```python
from build123d import *

# Parameters (mm, degrees)
SKETCH1_W           = 18.5
SKETCH1_H           = 40
BOSS_EXTRUDE1_DEPTH = 3
SKETCH2_W           = 1.5
SKETCH2_H           = 17.1
BOSS_EXTRUDE2_DEPTH = 60.5
CUT_EXTRUDE1_REACH  = 79.295
SKETCH4_W           = 15.5
SKETCH4_H           = 10.9


with BuildPart() as part:
    # Sketch1 → Boss-Extrude1 (new body)
    with BuildSketch(Plane(origin=(0, 0, 0), x_dir=(1, 0, 0), z_dir=(0, 1, 0))):
        with Locations((9.25, 20)):
            Rectangle(SKETCH1_W, SKETCH1_H)
    extrude(amount=BOSS_EXTRUDE1_DEPTH)

    # Sketch2 → Boss-Extrude2 (add)
    with BuildSketch(Plane(origin=(0, 3, 0), x_dir=(1, 0, 0), z_dir=(0, 1, 0))):
        Polygon((18.5, 40), (0, 40), (0, 37.1), (1.5, 37.1), (18.5, 37.1), align=None)
        Polygon((1.5, 37.1), (0, 37.1), (0, 0), (1.5, 0), (1.5, 2.9), align=None)
        Polygon((17, 2.9), (1.5, 2.9), (1.5, 0), (18.5, 0), (18.5, 2.9), align=None)
        with Locations((17.75, 11.45)):
            Rectangle(SKETCH2_W, SKETCH2_H)
    extrude(amount=BOSS_EXTRUDE2_DEPTH)

    # Sketch4 → Cut-Extrude1 (cut, up to next)
    with BuildSketch(Plane(origin=(0, 0, -40), x_dir=(-1, 0, 0), z_dir=(0, 0, -1)), mode=Mode.PRIVATE) as cut_extrude1_sk1:
        with Locations((-9.25, 8.45)):
            Rectangle(SKETCH4_W, SKETCH4_H)
    cut_extrude1_tool1 = extrude(cut_extrude1_sk1.sketch, amount=-CUT_EXTRUDE1_REACH, mode=Mode.PRIVATE) & part.part
    add(cut_extrude1_tool1.solids().sort_by_distance((9.25, 8.45, -40))[0], mode=Mode.SUBTRACT)


solid = part.part
```
Model file for the job. Use its own axes, mm. A direction names the side the tool comes from. Coordinates: 2 decimals unless noted, no trailing zeros. Order: outer loops, then holes, each group sorted by start corner. A loop starts at its lowest first (then second) coordinate and runs counter-clockwise, first axis right, second up. Notation, with made-up numbers: M 64,25.25 L 121,25.25 A16 cw 121,47.25 Z; hole C 33.25,83 d8. An arc over 180 degrees is marked long. Answer as CSV lines item,"result".
(1) Band-saw the part on B-B, the plane x = 4.25. List the corners of the cut face in (y, z), then the cut area to 3 significant figures.
Geometry says:
outline,"M 0,-40 L 3,-40 L 3,-2.9 L 63.5,-2.9 L 63.5,0 L 0,0 Z; M 13.9,-40 L 63.5,-40 L 63.5,-37.1 L 13.9,-37.1 Z"
area,"439 mm2"
(2) Wall check: line 1 along Z through (x, y) = (9.5, 57.5); line 2 along X through (y, z) = (29, -17); line 3 along X through (y, z) = (37, -30.5). Give the ranges that are in metal, low to high.
Geometry says:
line 1,"z = -40 to -37.1, -2.9 to 0"
line 2,"x = 0 to 1.5, 17 to 18.5"
line 3,"x = 0 to 1.5"
(3) Pull direction X, two halves, no side cores. Call faces 4 (the flat face through (9, 31, 0)), 5 (the flat face through (17, 33, -11)), 6 (the flat face through (9, 13.9, -39)), 7 (the flat face through (18.5, 31, -15)): +X half, -X half, draft (parallel to the pull), parting line (faces both ways), or undercut.
Geometry says:
face 4,"draft"
face 5,"undercut"
face 6,"undercut"
face 7,"+X half"
(4) Band-saw the part on A-A, the plane y = 9.5. List the corners of the cut face in (x, z), then the cut area to 3 significant figures.
Geometry says:
outline,"M 0,-40 L 1.5,-40 L 1.5,-2.9 L 17,-2.9 L 17,-20 L 18.5,-20 L 18.5,0 L 0,0 Z; M 17,-40 L 18.5,-40 L 18.5,-37.1 L 17,-37.1 Z"
area,"139 mm2"
(5) Flat gauge pin, fed straight in: pin 1 (5 mm diameter, centred on x = 13.5, z = -18, fed in from +Y). Where does the tip first touch, or does it go through?
Geometry says:
pin 1,"stops at y = 3"
(6) Band-saw the part on D-D, the plane y = 47. List the corners of the cut face in (x, z).
Geometry says:
outline,"M 0,-40 L 18.5,-40 L 18.5,-37.1 L 1.5,-37.1 L 1.5,-2.9 L 17,-2.9 L 17,-20 L 18.5,-20 L 18.5,0 L 0,0 Z"
(7) Band-saw the part on C-C, the plane z = -9. List the corners of the cut face in (x, y), then the cut area to 3 significant figures.
Geometry says:
outline,"M 0,0 L 18.5,0 L 18.5,63.5 L 17,63.5 L 17,3 L 1.5,3 L 1.5,63.5 L 0,63.5 Z"
area,"237 mm2"
(8) 3-axis set-ups, long thin cutter, end or side, ignore diameter. For faces 1 (the flat face through (18, 33, -20)), 2 (the flat face through (9, 33, -2.9)), 3 (the flat face through (17, 8, -39)): which of +Z, -Z, +X, -X, +Y, -Y reach the whole face in a straight line?
Geometry says:
face 1,"+X, +Y"
face 2,"+Y"
face 3,"-Z"
